The listing builds one solid part. Answer for the finished solid, in the listing's coordinates (mm). A direction names the side the tool comes from. Give positions to 0.01 mm unless a question says otherwise; leave off trailing zeros. Loops run counter-clockwise (first coordinate to the right, second up) from the corner with the lowest first, then second, coordinate; pieces in that order, holes last.
Item 1: A tool of negligible diameter and unlimited length cuts with its end or side. For faces 4 (the face through (-4.4, 3, 3.2)), 5 (the face through (-6.317, -0.093, 0.056)), 6 (the face through (-5, -16, 0)), 7 (the face through (5, 6, 0)), 8 (the face through (-3, -27.2, 0)), from which of +Z, -Z, +X, -X, +Y, -Y can it reach the whole face along a straight path? Write none if from no direction.
Item 2: Section A-A, the plane x = -2.5 is taken. Give the vertices of the cut face in (y, z).
Item 3: Section B-B, the plane z = 3 is taken. Give the vertices of the cut face in (x, y), and give its area (3 significant figures).
Item 4: Section C-C, the plane x = -14.5 is taken. Give the vertices of the cut face in (y, z).
Item 5: This flat-tipped pin is pushed along its axis until it touches: pin 1 Ø2 at (x, z) = (-12, 1.5) entering from +Y. Where does it stop, or does it pass through?
Item 6: Consider line 1 along Y through (x, z) = (-1.5, 2.25); line 2 along X through (y, z) = (-17, -0.75); line 3 along X through (y, z) = (-20.5, -1.5). Determine where each line is inside the solid, lowest interval first.
Item 7: The mould has two halves that part along Y. Classify faces 1 (the face through (8, -27, 0)), 2 (the face through (-5, 8, 0)), 3 (the face through (-3, -16.7, 0)): pulls with the +Y half, pulls with the -Y half, needs draft (parallel to the pull), parting line crosses it, or undercut.
Item 8: Section D-D, the plane y = 9 is taken. Give the vertices of the cut face in (x, z), and give its area (3 significant figures).
from build123d import *

# Parameters (mm, degrees)
CROQUIS1_R              = 5
SALIENTE_EXTRUIR1_DEPTH = 3
SALIENTE_EXTRUIR2_DEPTH = 4
CROQUIS4_R              = 5
SALIENTE_EXTRUIR3_DEPTH = 15
CROQUIS6_R              = 5
SALIENTE_EXTRUIR5_DEPTH = 20
CROQUIS3_R              = 5
SALIENTE_EXTRUIR7_DEPTH = 10
CROQUIS12_R             = 6
SALIENTE_EXTRUIR8_DEPTH = 12
CROQUIS11_W             = 60
CROQUIS11_H             = 5
CORTAR_EXTRUIR4_DEPTH   = 42


with BuildPart() as part:
    # Croquis1 → Saliente-Extruir1 (new body)
    with BuildSketch(Plane(origin=(0, 0, 0), x_dir=(1, 0, 0), z_dir=(0, 1, 0))):
        Circle(CROQUIS1_R)
    extrude(amount=SALIENTE_EXTRUIR1_DEPTH)

    # Croquis2 → Saliente-Extruir2 (add, symmetric)
    with BuildSketch(Plane.XY):
        Polygon((-5, 3), (-13, 2.43295135), (-17.863199041, -8.537431282), (-8.325792195, -25), (-1.391615301, -25), (-11.139227196, -8.174595228), (-7.597010616, -0.184078921), (-5, 0), (0, 0), (0, 3), align=None)
    extrude(amount=SALIENTE_EXTRUIR2_DEPTH, both=True)

    # Croquis4 → Saliente-Extruir3 (add)
    with BuildSketch(Plane(origin=(0, 0, 0), x_dir=(0, 0, -1), z_dir=(1, 0, 0))):
        with Locations((0, -22)):
            Circle(CROQUIS4_R)
    extrude(amount=-SALIENTE_EXTRUIR3_DEPTH)

    # Croquis6 → Saliente-Extruir5 (add)
    with BuildSketch(Plane(origin=(0, 0, 0), x_dir=(0, 0, -1), z_dir=(1, 0, 0))):
        with Locations((0, -22)):
            Circle(CROQUIS6_R)
    extrude(amount=SALIENTE_EXTRUIR5_DEPTH)

    # Croquis3 → Saliente-Extruir7 (add)
    with BuildSketch(Plane(origin=(0, 3, 0), x_dir=(1, 0, 0), z_dir=(0, 1, 0))):
        Circle(CROQUIS3_R)
    extrude(amount=SALIENTE_EXTRUIR7_DEPTH)

    # Croquis12 → Saliente-Extruir8 (add)
    with BuildSketch(Plane.ZY.offset(15)):
        with Locations((0, -22)):
            Circle(CROQUIS12_R)
    extrude(amount=-SALIENTE_EXTRUIR8_DEPTH)

    # Croquis11 → Cortar-Extruir4 (cut, through all)
    with BuildSketch(Plane(origin=(0, 13, 0), x_dir=(1, 0, 0), z_dir=(0, 1, 0))):
        with Locations((-3, 6.5)):
            Rectangle(CROQUIS11_W, CROQUIS11_H)
        with Locations((-3, -6.5)):
            Rectangle(CROQUIS11_W, CROQUIS11_H)
    extrude(amount=-CORTAR_EXTRUIR4_DEPTH, mode=Mode.SUBTRACT)


solid = part.part
Worked answers:
1. face 4: +Z, -X, +Y
1. face 5: +Z, -Z, +X
1. face 6: +X
1. face 7: +X, +Y
1. face 8: +X, -Y
2. outline: (-25, -4) - (-19, -4) arc R5 ccw to (-19, 4) - (-25, 4) arc R5 ccw to start; (0, -4) - (13, -4) - (13, 4) - (0, 4) - close
3. outline: (-17.86, -8.54) - (-13.07, -16.8) - (-15, -16.8) - (-15, -27.2) - (-3, -27.2) - (-3, -26) - (20, -26) - (20, -18) - (-3, -18) - (-3, -16.8) - (-6.14, -16.8) - (-11.14, -8.17) - (-7.6, -0.18) - (-5, 0) - (4, 0) - (4, 13) - (-4, 13) - (-4, 3) - (-5, 3) - (-13, 2.43) - close
3. area: 552 mm2
4. outline: (-26.47, -4) - (-17.53, -4) arc R6 ccw to (-17.53, 4) - (-26.47, 4) arc R6 ccw to start; (-14.34, -4) - (-0.95, -4) - (-0.95, 4) - (-14.34, 4) - close
5. pin 1: stops at y = 2.57
6. line 1: y = -26.47 to -17.53, 0 to 13
6. line 2: x = -15 to -3
6. line 3: x = -15 to 20
7. face 1: pulls with the -Y half
7. face 2: needs draft
7. face 3: undercut
8. outline: (-3, -4) - (3, -4) arc R5 ccw to (3, 4) - (-3, 4) arc R5 ccw to start
8. area: 70.4 mm2
